Check sheet for the modelled part. Datum: model origin and axes. Units: mm. Coordinates: 2 decimals unless noted, no trailing zeros. Loops run counter-clockwise (first coordinate to the right, second up) from the corner with the lowest first, then second, coordinate; pieces in that order, holes last. Notation, with made-up numbers: (-36, -31) -> (-1, -31) arc R14 ccw to (-1, -27) -> close; hole circle Ø10 at (19, -11). An arc over 180 degrees is marked (long way). Use CSV: the item, a comma, the result in double quotes.
```python
from build123d import *

# Parameters (mm, degrees)
SKETCH1_R           = 3.175
BOSS_EXTRUDE1_DEPTH = 6.35
SKETCH2_R           = 3.175
CUT_EXTRUDE1_DEPTH  = 118.260276735


with BuildPart() as part:
    # Sketch1 → Boss-Extrude1 (new body)
    with BuildSketch(Plane.XY):
        with BuildLine():
            Line((0, 0), (0, 101.6))
            ThreePointArc((0, 101.6), (12.7, 114.3), (25.4, 101.6))
            Line((25.4, 101.6), (25.4, 0))
            Line((25.4, 0), (0, 0))
        make_face()
        with Locations((12.7, 101.6)):
            Circle(SKETCH1_R, mode=Mode.SUBTRACT)
    extrude(amount=BOSS_EXTRUDE1_DEPTH)

    # Sketch2 → Cut-Extrude1 (cut, through all)
    with BuildSketch(Plane.XY.offset(6.35)):
        with Locations((12.7, 63.5)):
            Circle(SKETCH2_R)
        with Locations((12.7, 12.7)):
            Circle(SKETCH2_R)
    extrude(amount=-CUT_EXTRUDE1_DEPTH, mode=Mode.SUBTRACT)


solid = part.part
```
1) Cross-section at B-B on y = 12.7. Record the boundary of the cut face in (x, z) (3 decimals), and give its area (3 significant figures).
Answer below:
outline,"(0, 0) -> (9.525, 0) -> (9.525, 6.35) -> (0, 6.35) -> close; (15.875, 0) -> (25.4, 0) -> (25.4, 6.35) -> (15.875, 6.35) -> close"
area,"121 mm²"
2) Cross-section at C-C on x = 12.7. Record the boundary of the cut face in (y, z) (3 decimals), and give its area (3 significant figures).
Answer below:
outline,"(0, 0) -> (9.525, 0) -> (9.525, 6.35) -> (0, 6.35) -> close; (15.875, 0) -> (60.325, 0) -> (60.325, 6.35) -> (15.875, 6.35) -> close; (66.675, 0) -> (98.425, 0) -> (98.425, 6.35) -> (66.675, 6.35) -> close; (104.775, 0) -> (114.3, 0) -> (114.3, 6.35) -> (104.775, 6.35) -> close"
area,"605 mm²"
3) Draft check along X on faces 1 (the cylindrical face through (10.36, 65.646, 3.219)), 2 (the flat face through (25.4, 52, 3)), 3 (the flat face through (13, 58, 6.35)). Enter one of: released by +X, released by -X, zero draft, split by the parting line, or undercut.
Answer below:
face 1,"undercut"
face 2,"released by +X"
face 3,"zero draft"
4) Go/stop test with a flat-tipped pin: pin 1 Ø8.5 at (x, y) = (12.7, 101.6) entering from -Z. Record where the tip stops, or that it passes through.
Answer below:
pin 1,"stops at z = 0"
5) Cross-section at A-A on z = 3.25. Record the boundary of the cut face in (x, y) (3 decimals).
Answer below:
outline,"(0, 0) -> (25.4, 0) -> (25.4, 101.6) arc R12.7 ccw to (0, 101.6) -> close; hole circle Ø6.35 at (12.7, 12.7); hole circle Ø6.35 at (12.7, 63.5); hole circle Ø6.35 at (12.7, 101.6)"
6) Thickness scan on line 1 along Y through (x, z) = (12.7, 3) (3 decimals); line 2 along Y through (x, z) = (12, 2.5); line 3 along X through (y, z) = (104.5, 3.75). Record the ranges inside material, lowest first. Write a range as from..to.
Answer below:
line 1,"y = 0..9.525, 15.875..60.325, 66.675..98.425, 104.775..114.3"
line 2,"y = 0..9.6, 15.8..60.4, 66.6..98.5, 104.7..114.28"
line 3,"x = 0.34..11.41, 13.99..25.06"
